Verification items for this drawing (mm, ordinates from the low corner). A direction names the side the tool comes from. Coordinates: 2 decimals unless noted, no trailing zeros. Order: outer loops, then holes, each group sorted by start corner. A loop starts at its lowest first (then second) coordinate and runs counter-clockwise, first axis right, second up. Notation, with made-up numbers: M 82,-7 L 99,-7 A21 ccw 99,5 Z; hole C 15,7 d5. An arc over 180 degrees is marked long. Write item = value, one per line.
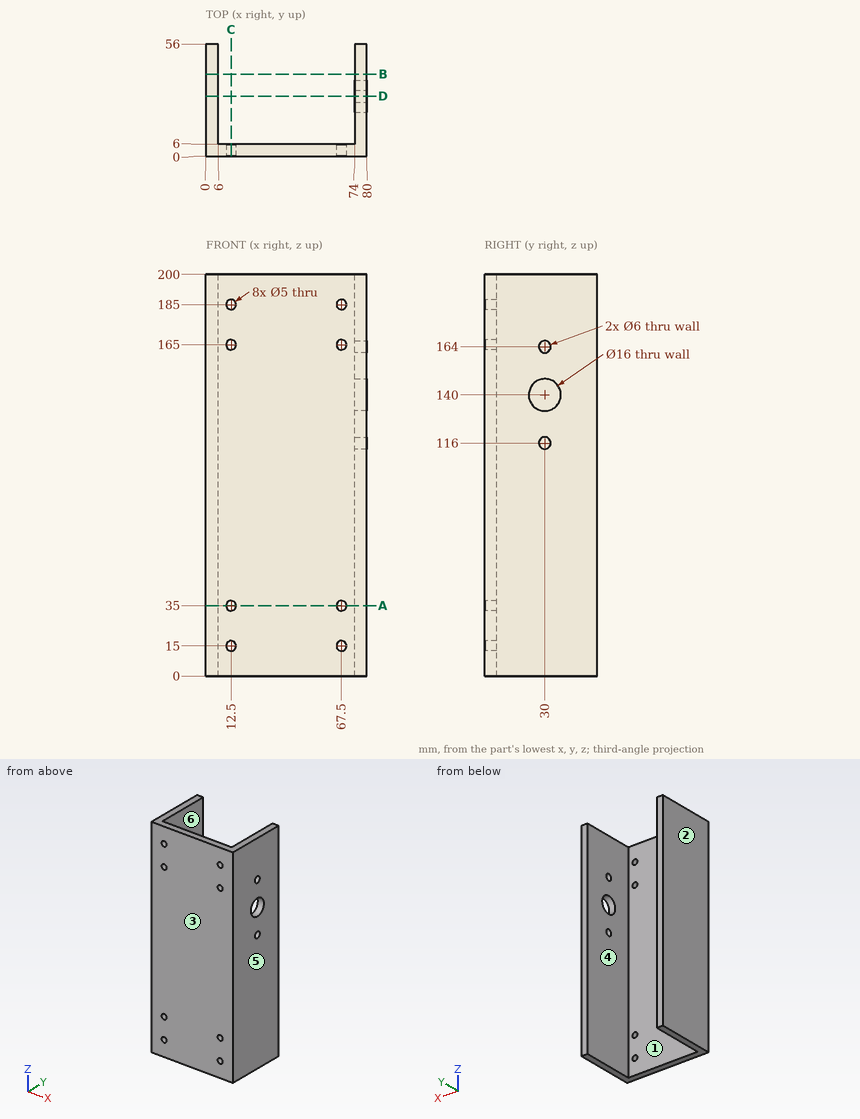
Item 1: Scan lines: L1, parallel to Z at x = 67.5, y = 3.3; L2, parallel to X at y = 3.2, z = 165; L3, parallel to X at y = 19, z = 121. Record each from-to range of solid material in increasing order. Write a range as from..to.
Report:
L1 = 0..12.5, 17.5..32.5, 37.5..162.5, 167.5..182.5, 187.5..200
L2 = 0..10, 15..65, 70..80
L3 = 0..6, 74..80
Item 2: Sectioned sample at C-C, the plane x = 12.5. Enter the section's corners in (y, z).
Report:
outline = M 0,0 L 6,0 L 6,12.5 L 0,12.5 Z; M 0,17.5 L 6,17.5 L 6,32.5 L 0,32.5 Z; M 0,37.5 L 6,37.5 L 6,162.5 L 0,162.5 Z; M 0,167.5 L 6,167.5 L 6,182.5 L 0,182.5 Z; M 0,187.5 L 6,187.5 L 6,200 L 0,200 Z
Item 3: Sectioned sample at B-B, the plane y = 41. Enter the section's corners in (x, z), then the cut area to 3 significant figures.
Report:
outline = M 0,0 L 6,0 L 6,200 L 0,200 Z; M 74,0 L 80,0 L 80,200 L 74,200 Z
area = 2,400 mm^2
Item 4: Release check for a two-part mould opening along X. For the marked faces 1, 2, 3 and 4 record: pulls with the +X half, pulls with the -X half, needs draft (parallel to the pull), parting line crosses it, or undercut.
Report:
face_1 = undercut
face_2 = pulls with the -X half
face_3 = needs draft
face_4 = undercut
Item 5: Sectioned sample at D-D, the plane y = 30. Enter the section's corners in (x, z).
Report:
outline = M 0,0 L 6,0 L 6,200 L 0,200 Z; M 74,0 L 80,0 L 80,113 L 74,113 Z; M 74,119 L 80,119 L 80,132 L 74,132 Z; M 74,148 L 80,148 L 80,161 L 74,161 Z; M 74,167 L 80,167 L 80,200 L 74,200 Z
Item 6: Gauge pin test, flat ends, axial feed: pin 1 (1 mm diameter, centred on x = 52.5, z = 96.5, fed in from +Y); pin 2 (13 mm diameter, centred on y = 30, z = 140, fed in from +X). Record the tip position at first contact, or that the pin passes through.
Report:
pin_1 = 6
pin_2 = 6
Item 7: Tool access check on the marked faces 5 and 6. Record the directions out of +Z, -Z, +X, -X, +Y, -Y that give a thin tool (end or side, any length) a straight path to the whole face; none if there is none.
Report:
face_5 = +Z, -Z, +X, +Y, -Y
face_6 = +Z, -Z, +Y
Item 8: Sectioned sample at A-A, the plane z = 35. Enter the section's corners in (x, y), then the cut area to 3 significant figures.
Report:
outline = M 0,0 L 10,0 L 10,6 L 6,6 L 6,56 L 0,56 Z; M 15,0 L 65,0 L 65,6 L 15,6 Z; M 70,0 L 80,0 L 80,56 L 74,56 L 74,6 L 70,6 Z
area = 1,020 mm^2
